Part model, mm, in its own coordinate system. Round coordinates to 2 decimals unless told otherwise and drop trailing zeros. Write each loop counter-clockwise with the first axis right and the second up, starting at its lowest first coordinate (ties: lowest second). Pieces come first, ordered by that corner, then holes. Notation, with made-up numbers: (7.25, 51) -> (54.25, 51) arc R15 cw to (54.25, 56) -> close; hole circle Ø8 at (69.5, 85). An arc over 180 degrees is marked (long way). Return JSON: item names as keys, results as strings. Group by question number.
(1) Saw through at D-D (x = -1.5). List the corners of the cut face in (y, z).
(2) Drill centre lines: L1, parallel to X at y = -15, z = 1.5; L2, parallel to Y at x = -26.5, z = 2; L3, parallel to X at y = -16.5, z = 5.5. Where is each one in solid material? Low to high. Write a range as from..to.
(3) Saw through at B-B (z = 1.25). State how many separate pieces and enclosed holes the cut face has, plus the area to 3 significant figures.
(4) Saw through at A-A (x = -17.5). List the corners of the cut face in (y, z).
(5) Saw through at C-C (x = 15). List the corners of the cut face in (y, z), plus the area to 3 significant figures.
(6) Mould opens along Y. For faces 1 (the flat face through (-7, 0, 0)), 2 (the cylindrical face through (13.7, -16.2, 3.2)), 3 (the flat face through (-7, -19.05, 3)) say: +Y half, -Y half, draft (parallel to the pull), parting line (faces both ways), or undercut.
from build123d import *

# Parameters (mm, degrees)
SKETCH1_W           = 50.8
SKETCH1_H           = 38.1
BOSS_EXTRUDE1_DEPTH = 6.35
SKETCH2_R           = 2.38125
SKETCH2_R_2         = 4.7625
CUT_EXTRUDE1_DEPTH  = 38.567106623
SKETCH3_R           = 1.778
CUT_EXTRUDE2_DEPTH  = 38.567106623


with BuildPart() as part:
    # Sketch1 → Boss-Extrude1 (new body)
    with BuildSketch(Plane.XY):
        with Locations((-6.35, 0)):
            Rectangle(SKETCH1_W, SKETCH1_H)
    extrude(amount=BOSS_EXTRUDE1_DEPTH)

    # Sketch2 → Cut-Extrude1 (cut, through all)
    with BuildSketch(Plane.XY.offset(6.35)):
        with Locations((-17.462302917, 0.082964446)):
            Circle(SKETCH2_R)
        Circle(SKETCH2_R_2)
    extrude(amount=-CUT_EXTRUDE1_DEPTH, mode=Mode.SUBTRACT)

    # Sketch3 → Cut-Extrude2 (cut, through all)
    with BuildSketch(Plane.XY.offset(6.35)):
        with Locations((-27.78125, 15.08125)):
            Circle(SKETCH3_R)
        with Locations((15.08125, 15.08125)):
            Circle(SKETCH3_R)
        with Locations((15.08125, -15.08125)):
            Circle(SKETCH3_R)
        with Locations((-27.78125, -15.08125)):
            Circle(SKETCH3_R)
    extrude(amount=-CUT_EXTRUDE2_DEPTH, mode=Mode.SUBTRACT)


solid = part.part
Computed values:
{
 "1": {"outline": "(-19.05, 0) -> (-4.52, 0) -> (-4.52, 6.35) -> (-19.05, 6.35) -> close; (4.52, 0) -> (19.05, 0) -> (19.05, 6.35) -> (4.52, 6.35) -> close"},
 "2": {"L1": "-31.75..-29.56, -26.01..13.31, 16.86..19.05", "L2": "-19.05..-16.31, -13.85..13.85, 16.31..19.05", "L3": "-31.75..-28.85, -26.71..14.01, 16.15..19.05"},
 "3": {"separate pieces": "1", "enclosed holes": "6", "area": "1,810 mm2"},
 "4": {"outline": "(-19.05, 0) -> (-2.3, 0) -> (-2.3, 6.35) -> (-19.05, 6.35) -> close; (2.46, 0) -> (19.05, 0) -> (19.05, 6.35) -> (2.46, 6.35) -> close"},
 "5": {"outline": "(-19.05, 0) -> (-16.86, 0) -> (-16.86, 6.35) -> (-19.05, 6.35) -> close; (-13.31, 0) -> (13.31, 0) -> (13.31, 6.35) -> (-13.31, 6.35) -> close; (16.86, 0) -> (19.05, 0) -> (19.05, 6.35) -> (16.86, 6.35) -> close", "area": "197 mm2"},
 "6": {"face 1": "draft", "face 2": "undercut", "face 3": "-Y half"}
}
